from build123d import *

# Parameters (mm, degrees)
SKETCH1_W                       = 300
SKETCH1_H                       = 50
BOSS_EXTRUDE1_DEPTH             = 30
F_8_0MM_DOWEL_HOLE1_D           = 8
F_8_0MM_DOWEL_HOLE1_CSINK_D     = 8.05
F_8_0MM_DOWEL_HOLE1_CSINK_ANGLE = 90


with BuildPart() as part:
    # Sketch1 → Boss-Extrude1 (new body)
    with BuildSketch(Plane.XY):
        with Locations((150, 25)):
            Rectangle(SKETCH1_W, SKETCH1_H)
    extrude(amount=BOSS_EXTRUDE1_DEPTH)

    # Ø8.0mm Dowel Hole1 (through all)
    with Locations(Plane.XY.offset(30)):
        with Locations((10, 37.5)):
            CounterSinkHole(F_8_0MM_DOWEL_HOLE1_D / 2, F_8_0MM_DOWEL_HOLE1_CSINK_D / 2, counter_sink_angle=F_8_0MM_DOWEL_HOLE1_CSINK_ANGLE)


solid = part.part
Geometry: final body of the model. Coordinates: model frame, mm. Coordinates: 2 decimals unless noted, no trailing zeros. Loops run counter-clockwise (first coordinate to the right, second up) from the corner with the lowest first, then second, coordinate; pieces in that order, holes last. Notation, with made-up numbers: M -10.75,35 L 33.25,35 A18 cw 33.25,66 Z; hole C 54,69 d7. An arc over 180 degrees is marked long. One line per item, written item: value. Start each with the question number.
1) Cut plane B-B (y = 37.5). Return loops of the section in (x, z) (3 decimals), then the cut area to 3 significant figures.
2) Cut plane A-A (x = 10). Return loops of the section in (y, z) (3 decimals), then the cut area to 3 significant figures.
3) Draft query along X for faces 1 (the flat face through (148, 0, 15)), 2 (the cylindrical face through (10.521, 41.466, 14.778)), 3 (the flat face through (0, 25, 15)). Return one class per face: released by +X, released by -X, zero draft, split by the parting line, or undercut.
4) Material intervals for L1, parallel to Y at x = 10, z = 12; L2, parallel to X at y = 37.5, z = 8.75; L3, parallel to X at y = 36, z = 18, sorted ascending. Write a range as from..to.
Evaluation:
1. outline: M 0,0 L 6,0 L 6,29.975 L 5.975,30 L 0,30 Z; M 14,0 L 300,0 L 300,30 L 14.025,30 L 14,29.975 Z
1. area: 8,760 mm^2
2. outline: M 0,0 L 33.5,0 L 33.5,29.975 L 33.475,30 L 0,30 Z; M 41.5,0 L 50,0 L 50,30 L 41.525,30 L 41.5,29.975 Z
2. area: 1,260 mm^2
3. face 1: zero draft
3. face 2: undercut
3. face 3: released by -X
4. L1: 0..33.5, 41.5..50
4. L2: 0..6, 14..300
4. L3: 0..6.29, 13.71..300
